CAD build for the part. Positions are in the model's coordinates, mm. Face numbers are marked on the shaded views. Coordinates: 2 decimals unless noted, no trailing zeros. Loops run counter-clockwise (first coordinate to the right, second up) from the corner with the lowest first, then second, coordinate; pieces in that order, holes last. Notation, with made-up numbers: (44.25, 72) -> (57.25, 72) arc R17 ccw to (57.25, 89) -> close; hole circle Ø8 at (-19.5, 49). An arc over 180 degrees is marked (long way). Answer as CSV lines item,"result". Start each with the question number.
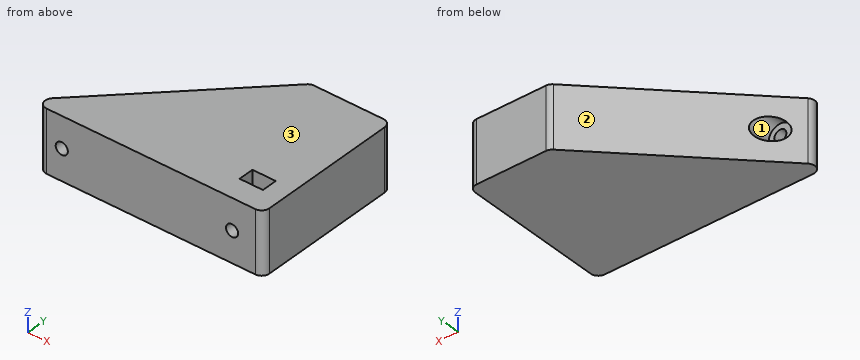
from build123d import *

# Parameters (mm, degrees)
BOSS_EXTRUDE1_DEPTH = 25.4
SKETCH3_R           = 2.4892
CUT_EXTRUDE1_DEPTH  = 25.4
SKETCH5_W           = 9.5758
SKETCH5_H           = 6.35
CUT_EXTRUDE2_DEPTH  = 17.5133
SKETCH7_R           = 4.7879
CUT_EXTRUDE3_DEPTH  = 54.61
FILLET3_R           = 3.175


with BuildPart() as part:
    # Sketch1 → Boss-Extrude1 (new body)
    with BuildSketch(Plane.XY):
        Polygon((0, 0), (63.5, 63.5), (96.42348, 63.5), (96.42348, 0), align=None)
    extrude(amount=-BOSS_EXTRUDE1_DEPTH)

    # Sketch3 → Cut-Extrude1 (cut)
    with BuildSketch(Plane.XZ):
        with Locations((83.72348, -12.7)):
            Circle(SKETCH3_R)
        with Locations((13.87348, -12.7)):
            Circle(SKETCH3_R)
    extrude(amount=-CUT_EXTRUDE1_DEPTH, mode=Mode.SUBTRACT)

    # Sketch5 → Cut-Extrude2 (cut)
    with BuildSketch(Plane.XY):
        with Locations((83.72348, 12.7)):
            Rectangle(SKETCH5_W, SKETCH5_H)
    extrude(amount=-CUT_EXTRUDE2_DEPTH, mode=Mode.SUBTRACT)

    # Sketch7 → Cut-Extrude3 (cut)
    with BuildSketch(Plane(origin=(0, 63.5, 0), x_dir=(1, 0, 0), z_dir=(0, 1, 0))):
        with Locations(Location((13.87348, 12.7, 0), (0, 0, 270))):
            Circle(SKETCH7_R)
    extrude(amount=-CUT_EXTRUDE3_DEPTH, mode=Mode.SUBTRACT)

    # Fillet3
    fillet3_edges = [part.edges().sort_by_distance(p)[0] for p in [
        (0, 0, -12.7),
        (63.5, 63.5, -12.7),
        (96.42348, 63.5, -12.7),
        (96.42348, 0, -12.7),
    ]]
    fillet(fillet3_edges, radius=FILLET3_R)


solid = part.part
Item 1: Saw through at D-D (x = 51). Write the cut outline in (y, z).
Item 2: Two-plate mould, pull along Z, no slides. Class the marked faces 1, 2 and 3: pulls with the +Z half, pulls with the -Z half, needs draft (parallel to the pull), parting line crosses it, or undercut.
Item 3: Saw through at A-A (z = -12.7). Write the cut outline in (x, y) (3 decimals), plus the area to 3 significant figures.
Item 4: Saw through at C-C (y = 17.5). Write the cut outline in (x, z).
Item 5: Saw through at B-B (z = -3). Write the cut outline in (x, y) (3 decimals).
Item 6: Flat gauge pins, fed straight in: pin 1 Ø5 at (x, z) = (54.5, -3.5) entering from +Y; pin 2 Ø1.5 at (x, z) = (39.5, -4.5) entering from +Y; pin 3 Ø3 at (x, z) = (13.87, -12.7) entering from -Y; pin 4 Ø3 at (y, z) = (11.5, -12) entering from -X. Where does each tip first touch, or does it go through?
Item 7: Wall check: probe 1 along X at (y, z) = (14.5, -12.7); probe 2 along Y at (x, z) = (87.5, -9.5) (3 decimals); probe 3 along X at (y, z) = (12, -16.5). Give the ranges that are in metal, low to high.
Geometry check:
1,outline,"(0, -25.4) -> (51, -25.4) -> (51, 0) -> (0, 0) -> close"
2,face 1,"undercut"
2,face 2,"needs draft"
2,face 3,"pulls with the +Z half"
3,outline,"(5.42, 5.42) arc R3.175 ccw to (7.665, 0) -> (11.384, 0) -> (11.384, 8.89) -> (9.086, 8.89) -> (9.086, 9.086) -> close; (16.363, 0) -> (81.234, 0) -> (81.234, 9.525) -> (78.936, 9.525) -> (78.936, 15.875) -> (81.234, 15.875) -> (81.234, 25.4) -> (86.213, 25.4) -> (86.213, 15.875) -> (88.511, 15.875) -> (88.511, 9.525) -> (86.213, 9.525) -> (86.213, 0) -> (93.248, 0) arc R3.175 ccw to (96.423, 3.175) -> (96.423, 60.325) arc R3.175 ccw to (93.248, 63.5) -> (64.815, 63.5) arc R3.175 ccw to (62.57, 62.57) -> (18.661, 18.661) -> (18.661, 8.89) -> (16.363, 8.89) -> close"
3,area,"3,840 mm2"
4,outline,"(17.5, -25.4) -> (96.42, -25.4) -> (96.42, 0) -> (17.5, 0) -> (17.5, -9.57) arc R4.79 cw to (17.5, -15.83) -> close; hole circle Ø4.98 at (83.72, -12.7)"
5,outline,"(5.42, 5.42) arc R3.175 ccw to (7.665, 0) -> (93.248, 0) arc R3.175 ccw to (96.423, 3.175) -> (96.423, 60.325) arc R3.175 ccw to (93.248, 63.5) -> (64.815, 63.5) arc R3.175 ccw to (62.57, 62.57) -> close; hole (78.936, 9.525) -> (88.511, 9.525) -> (88.511, 15.875) -> (78.936, 15.875) -> close"
6,pin 1,"y = 57"
6,pin 2,"y = 40.25"
6,pin 3,"through"
6,pin 4,"x = 18.13"
7,probe 1,"18.66 to 78.94, 88.51 to 96.42"
7,probe 2,"0 to 9.525, 15.875 to 63.5"
7,probe 3,"16.79 to 78.94, 88.51 to 96.42"
